Can you work these out from the drawing? Everything is in mm from the part's minimum corner. Round coordinates to 2 decimals unless told otherwise and drop trailing zeros. Order: outer loops, then holes, each group sorted by start corner. A loop starts at its lowest first (then second) coordinate and runs counter-clockwise, first axis right, second up. Notation, with made-up numbers: M 62,39.25 L 74,39.25 A35 ccw 74,73.25 Z; hole C 55,51.25 d8. An arc over 180 degrees is marked long. Write item = value, one per line. Start each with the question number.
Item 1: Please list where these lines run through material, in increasing order: L1, parallel to Y at x = 57, z = 6.25; L2, parallel to X at y = 56, z = 7.5; L3, parallel to X at y = 94, z = 18.
Item 2: I want a section at B-B, the plane z = 19.75. List the corners of the cut face in (x, y) for me.
Item 3: I'm going to push flat-ended pins straight in: P1, Ø1, axis at x = 12.5, z = 14.5, coming from the +Y side; P2, Ø6, axis at x = 90, z = 19.5, coming from the +Y side (1 decimal); P3, Ø4, axis at y = 56, z = 13, coming from the -X side; P4, Ø1.5, axis at x = 71.5, z = 15, coming from the +Y side. Where does each tip first touch, or does it pass through?
Item 4: I want a section at A-A, the plane x = 57.15. List the corners of the cut face in (y, z) for me.
Item 5: I want a section at C-C, the plane y = 71.5. List the corners of the cut face in (x, z) for me (1 decimal).
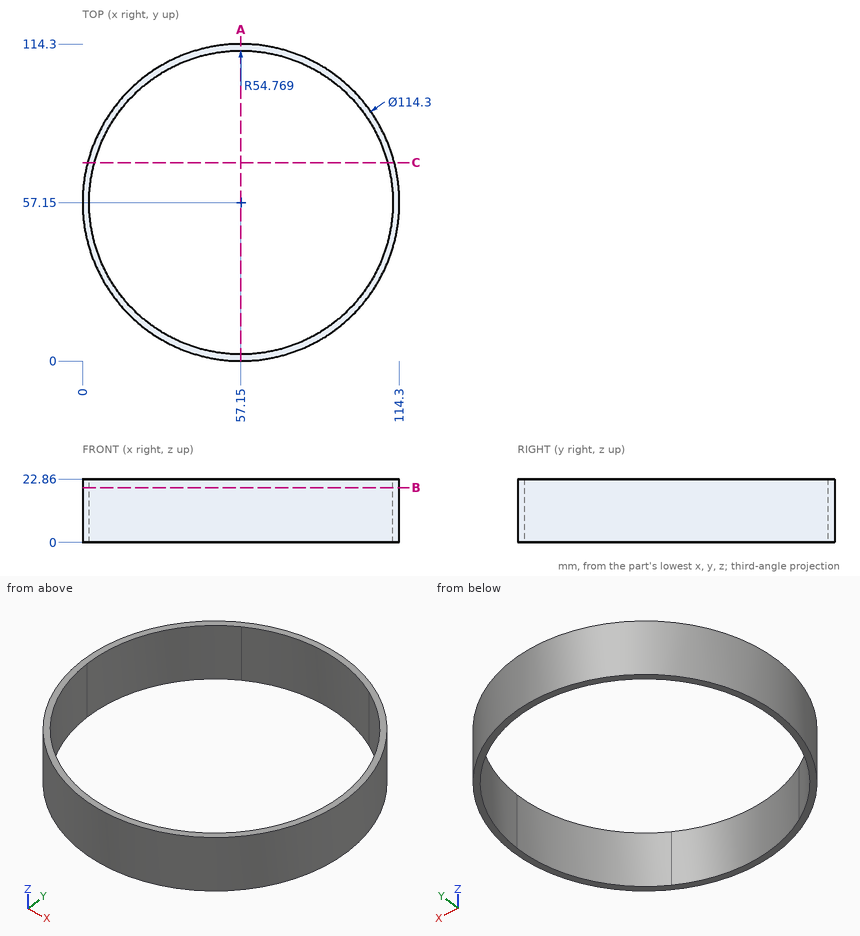
Filled in:
q1.L1 = 0 to 2.38, 111.92 to 114.3
q1.L2 = 0.01 to 2.39, 111.91 to 114.29
q1.L3 = 13.47 to 16.63, 97.67 to 100.83
q2.outline = C 57.15,57.15 d114.3; hole C 57.15,57.15 d109.54
q3.P1 = 93.44
q3.P2 = 105.9
q3.P3 = 0
q3.P4 = 112.66
q4.outline = M 0,0 L 2.38,0 L 2.38,22.86 L 0,22.86 Z; M 111.92,0 L 114.3,0 L 114.3,22.86 L 111.92,22.86 Z
q5.outline = M 1.8,0 L 4.3,0 L 4.3,22.9 L 1.8,22.9 Z; M 110,0 L 112.5,0 L 112.5,22.9 L 110,22.9 Z
